Autodesk Inventor part; units mm, degrees
ref_plane "YZ Plane" through (0, 0, 0) normal (1, 0, 0) x (0, 1, 0)
ref_plane "XZ Plane" through (0, 0, 0) normal (0, 1, 0) x (-1, 0, 0)
ref_plane "XY Plane" through (0, 0, 0) normal (0, 0, 1) x (1, 0, 0)
sketch "Sketch1" plane through (0, 0, 0) normal (0, 1, 0) x (-1, 0, 0)
  circle A0 centre (0, 0) radius 4.7625
  dimension "d0" = 9.525
extrude "Extrusion1" add sketch "Sketch1" along normal blind 101.6
chamfer "Chamfer1" distance 1.27 angle 45 1 edges at (4.7625, 101.6, 0)
chamfer "Chamfer2" distance 1.27 angle 45 1 edges at (4.7625, 0, 0)
properties part number "38shaft"
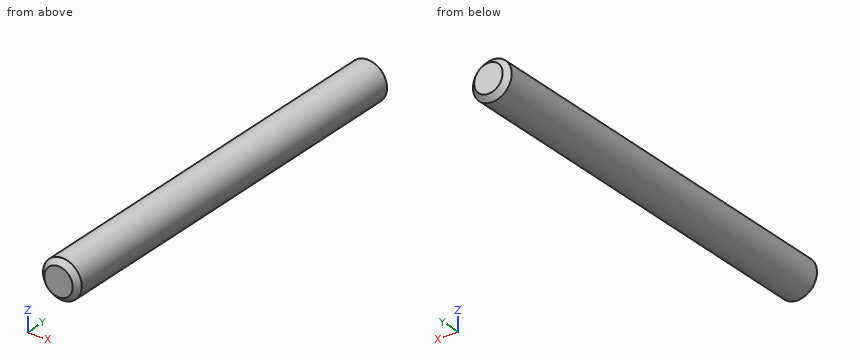
Geometry: final body of the model. Coordinates: model frame, mm. Round coordinates to 2 decimals unless told otherwise and drop trailing zeros. Order: outer loops, then holes, each group sorted by start corner. A loop starts at its lowest first (then second) coordinate and runs counter-clockwise, first axis right, second up. Notation, with made-up numbers: (11, 8.5) -> (59, 8.5) arc R30 ccw to (59, 31.5) -> close; hole circle Ø4 at (33.25, -22.5). An arc over 180 degrees is marked (long way). Use one line per item in the form item = value. Start each with the question number.
1. Line query: probe 1 along Z at (x, y) = (-0.25, 52); probe 2 along X at (y, z) = (8.5, 3.25); probe 3 along Y at (x, z) = (3.5, -2.25). Output: solid intervals per line, ascending.
2. Cut plane A-A (y = 60). Return the cut outline in (x, z) (1 decimal).
3. Pin query (flat end, axial travel): pin 1 Ø3 at (y, z) = (84.5, -2) entering from +X; pin 2 Ø3 at (x, y) = (-2.5, 90) entering from +Z; pin 3 Ø1 at (x, y) = (2.5, 79) entering from +Z. Return the tip coordinate at first contact, or that it passes through.
Solution:
q1.probe_1 = -4.76 to 4.76
q1.probe_2 = -3.48 to 3.48
q1.probe_3 = 0.67 to 100.93
q2.outline = circle Ø9.5 at (0, 0)
q3.pin_1 = 4.74
q3.pin_2 = 4.66
q3.pin_3 = 4.32
